Geometry check sheet. Reference: the model listing, model coordinates, mm. A direction names the side the tool comes from. Give positions to 0.01 mm unless a question says otherwise; leave off trailing zeros. Loops run counter-clockwise (first coordinate to the right, second up) from the corner with the lowest first, then second, coordinate; pieces in that order, holes last.
1. Tool access check on faces 1 (the flat face through (4, -4, 2.5)), 2 (the cylindrical face through (-46, 0, 14)). Record the directions out of +Z, -Z, +X, -X, +Y, -Y that give a thin tool (end or side, any length) a straight path to the whole face; none if there is none.
2. Release check for a two-part mould opening along Y. For faces 3 (the cylindrical face through (-33.727, 25.861, 17.976)), 4 (the flat face through (10, 1, 0)), 5 (the cylindrical face through (0, -46, 14)), 6 (the cylindrical face through (-1.08, 4.88, 1.23)) record: +Y half, -Y half, draft (parallel to the pull), parting line (faces both ways), or undercut.
3. Cross-section at A-A, the plane x = 0. Record the cut outline in (y, z).
4. Cross-section at B-B, the plane y = -26. Record the cut outline in (x, z), plus the area to 3 significant figures.
5. Go/stop test with flat-tipped pins: pin 1 Ø9.5 at (x, y) = (15.31, -15.31) entering from +Z; pin 2 Ø4 at (y, z) = (-14, 24) entering from +X; pin 3 Ø14 at (x, y) = (-15.31, 15.31) entering from +Z; pin 4 Ø1.5 at (x, z) = (7, 12) entering from +Y. Record where each tip stops, or that it passes through.
6. Material ranges on L1, parallel to X at y = 10.5, z = 2; L2, parallel to Y at x = -33, z = 23; L3, parallel to Z at x = -27, y = -10, recorded low to high.
7. Cross-section at C-C, the plane z = 16.5. Record the cut outline in (x, y).
8. Cross-section at D-D, the plane x = 14. Record the cut outline in (y, z), plus the area to 3 significant figures.
Autodesk Inventor part; units mm, degrees
ref_plane "Work Plane2" through (46, 0, 28.75) normal (0.8365, -0.5, 0.2241) x (-0.2588, 0, 0.9659)
ref_plane "YZ Plane" through (0, 0, 0) normal (1, 0, 0) x (0, 1, 0)
ref_plane "XZ Plane" through (0, 0, 0) normal (0, 1, 0) x (-1, 0, 0)
sketch "Sketch1" plane through (0, 0, 0) normal (0, 0, 1) x (1, 0, 0)
  circle A0 centre (0, 0) radius 5
  circle A1 centre (0, 0) radius 8.45
  circle A2 centre (0, 0) radius 42.5
  circle A3 centre (0, 0) radius 45 construction
  circle A4 centre (-31.8198, 31.8198) radius 1.45
  arc A5 (-28.0933, 35.1535) -> (-35.1535, 28.0933) centre (-31.8198, 31.8198) ccw
  arc A6 (-35.1535, -28.0933) -> (-28.0933, -35.1535) centre (-31.8198, -31.8198) ccw
  circle A7 centre (-31.8198, -31.8198) radius 1.45
  arc A8 (28.0933, -35.1535) -> (35.1535, -28.0933) centre (31.8198, -31.8198) ccw
  circle A9 centre (31.8198, -31.8198) radius 1.45
  arc A10 (35.1535, 28.0933) -> (28.0933, 35.1535) centre (31.8198, 31.8198) ccw
  circle A11 centre (31.8198, 31.8198) radius 1.45
  line L0 (-31.8198, 31.8198) -> (31.8198, 31.8198) construction
  arc A12 (28.841, 35.8357) -> (-28.841, 35.8357) centre (0, 0) ccw
  arc A13 (-35.8357, 28.841) -> (-35.8357, -28.841) centre (0, 0) ccw
  arc A14 (-28.841, -35.8357) -> (28.841, -35.8357) centre (0, 0) ccw
  arc A15 (35.8357, -28.841) -> (35.8357, 28.841) centre (0, 0) ccw
  point P0 (0, -46)
  point P1 (0, 46)
  dimension "d2" = 10
  dimension "d3" = 16.9
  dimension "d4" = 85
  dimension "d5" = 90
  dimension "d6" = 2.9
  dimension "d7" = 5
  dimension "d8" = 360
  dimension "d9" = 92
extrude "Extrusion1" add sketch "Sketch1" along normal blind 2.5 contours A1
extrude "Extrusion2" add sketch "Sketch1" along normal blind 7.5 contours A2
extrude "Extrusion3" add sketch "Sketch1" along normal blind 28.75 contours A12 A10 A15 A8 A14 A6 A13 A5
sketch "Sketch2" plane through (0, 0, 28.75) normal (0, 0, 1) x (1, 0, 0)
  arc A0 (35.8357, -28.841) -> (35.8357, 28.841) centre (0, 0) ccw construction
  line L0 (46, 0) -> (46, -31.8198) construction
  point P0 (31.8198, -31.8198)
ref_plane "Work Plane1" through (46, 0, 28.75) normal (0.9659, 0, 0.2588) x (0, -1, 0)
sketch "Sketch3" plane through (46, 0, 28.75) normal (0.9659, 0, 0.2588) x (0, -1, 0)
  ellipse E0 centre (0, -11.9057) end of major axis (-46, -11.9057) minor radius 11.9057 (28.841, -2.6307) -> (-28.841, -2.6307) ccw
  line L0 (0, 0) -> (0, -11.9057) construction
  point P0 (0, 15.8647)
ref_plane "Work Plane2" through (46, 0, 28.75) normal (0.8365, -0.5, 0.2241) x (-0.2588, 0, 0.9659)
sketch "Sketch4" plane through (46, 0, 28.75) normal (0.8365, -0.5, 0.2241) x (-0.2588, 0, 0.9659)
  circle A0 centre (0, 0) radius 5.325
  point P0 (-15.8647, 25.9368)
  dimension "d18" = 10.65
extrude "Extrusion4" cut sketch "Sketch4" along normal mid plane 30
sketch "Sketch5" plane through (0, 0, 7.5) normal (0, 0, 1) x (1, 0, 0)
  circle A0 centre (0, 21.65) radius 6
  line L0 (0, 21.65) -> (0, 0)
  circle A1 centre (-15.3089, 15.3089) radius 6
  circle A2 centre (-21.65, 0) radius 6
  circle A3 centre (-15.3089, -15.3089) radius 6
  circle A4 centre (0, -21.65) radius 6
  circle A5 centre (15.3089, -15.3089) radius 6
  circle A6 centre (21.65, 0) radius 6
  circle A7 centre (15.3089, 15.3089) radius 6
  dimension "d21" = 12
  dimension "d22" = 21.65
  dimension "d25" = 360
extrude "Extrusion5" cut sketch "Sketch5" against normal through all
properties part number "Case Part 1 - V3"
Result:
1. face 1: +Z
1. face 2: +Z, -Z, -X
2. face 3: undercut
2. face 4: draft
2. face 5: -Y half
2. face 6: undercut
3. outline: (-46, 0) - (-27.65, 0) - (-27.65, 7.5) - (-42.5, 7.5) - (-42.5, 28.75) - (-46, 28.75) - close; (-15.65, 0) - (-5, 0) - (-5, 2.5) - (-8.45, 2.5) - (-8.45, 7.5) - (-15.65, 7.5) - close; (5, 0) - (15.65, 0) - (15.65, 7.5) - (8.45, 7.5) - (8.45, 2.5) - (5, 2.5) - close; (27.65, 0) - (46, 0) - (46, 28.75) - (42.5, 28.75) - (42.5, 7.5) - (27.65, 7.5) - close
4. outline: (-37.95, 0) - (-4.13, 0) - (-4.13, 7.5) - (-33.62, 7.5) - (-33.62, 28.75) - (-37.95, 28.75) - close; (4.13, 0) - (37.95, 0) - (37.95, 28.75) - (33.62, 28.75) - (33.62, 7.5) - (4.13, 7.5) - close
4. area: 691 mm2
5. pin 1: passes through
5. pin 2: stops at x = 44.41
5. pin 3: stops at z = 7.5
5. pin 4: stops at y = 45.57
6. L1: x = -44.79 to -18.9, -11.72 to 11.72, 18.9 to 44.79
6. L2: y = -36.68 to -32.66, -30.98 to -26.78, 26.78 to 30.98, 32.66 to 36.68
6. L3: z = 0 to 7.5
7. outline: (-35.84, -28.84) arc R5 ccw to (-28.84, -35.84) arc R46 ccw to (28.84, -35.84) arc R5 ccw to (35.84, -28.84) arc R46 ccw to (35.84, 28.84) arc R5 ccw to (28.84, 35.84) arc R46 ccw to (-28.84, 35.84) arc R5 ccw to (-35.84, 28.84) arc R46 ccw to start; hole circle Ø85 at (0, 0); hole circle Ø2.9 at (-31.82, -31.82); hole circle Ø2.9 at (-31.82, 31.82); hole circle Ø2.9 at (31.82, -31.82); hole circle Ø2.9 at (31.82, 31.82)
8. outline: (-43.82, 0) - (-21.16, 0) - (-21.16, 7.5) - (-40.13, 7.5) - (-40.13, 28.75) - (-43.82, 28.75) - close; (-9.45, 0) - (9.45, 0) - (9.45, 7.5) - (-9.45, 7.5) - close; (21.16, 0) - (43.82, 0) - (43.82, 28.75) - (40.13, 28.75) - (40.13, 7.5) - (21.16, 7.5) - close
8. area: 638 mm2
